The model under review builds one solid part; all positions refer to its coordinate system, in mm. A direction names the side the tool comes from. Round coordinates to 2 decimals unless told otherwise and drop trailing zeros. Write each loop counter-clockwise with the first axis right and the second up, starting at its lowest first coordinate (ties: lowest second). Pieces come first, ordered by that corner, then holes.
Item 1: Add section B-B (z = -13). Give the boundary of the cut face in (x, y), plus the area to 3 significant figures.
Item 2: Clearance check with flat-ended pins moving along their axes: pin 1 Ø3 at (y, z) = (-2.5, 20) entering from -X; pin 2 Ø3 at (x, y) = (-15.5, -4.5) entering from -Z (3 decimals); pin 3 Ø5.5 at (x, z) = (0, -14.29) entering from +Y; pin 4 Ø1.5 at (x, z) = (12, 20) entering from +Y. State where each tip first meets the part, or that it passes through.
Item 3: Machinability: for faces 1 (the face through (-12.7, -3, -8)), 2 (the face through (-6.45, -3, 28)), 3 (the face through (12.7, -3, -8)), 4 (the face through (12.7, -3, 21)), which of the approach directions +Z, -Z, +X, -X, +Y, -Y give a long, thin tool a straight path to every point of the face, cutting with its end or side? Answer none if there is none.
Item 4: Add section A-A (x = 0). Give the boundary of the cut face in (y, z) (1 decimal).
Item 5: Add section D-D (x = -7.5). Give the boundary of the cut face in (y, z) (3 decimals), plus the area to 3 significant figures.
Item 6: To check wall thickness, follow L1, parallel to Z at x = 0, y = -3.85 (1 decimal); L2, parallel to X at y = -4.05, z = 21; L3, parallel to Z at x = -1.5, y = -3.3 (3 decimals). State the ranges of each line that lie inside material, in increasing order.
```python
from build123d import *

# Parameters (mm, degrees)
F0_R     = 3.175
F1_DEPTH = 5.842
F2_R     = 3.175


with BuildPart() as f1:
    # F0 (on Front) → F1 (new body)
    with BuildSketch(Plane.XZ):
        Polygon((-6.45, 25.4), (-12.7, 25.4), (-12.7, 15.875), (-18.542, 15.875), (-18.542, 3.175), (-12.7, 3.175), (-12.7, -6.35), (-12.7, -22.225), (12.7, -22.225), (12.7, -6.35), (12.7, 3.175), (18.542, 3.175), (18.542, 15.875), (12.7, 15.875), (12.7, 25.4), (6.45, 25.4), (6.45, 31.242), (-6.45, 31.242), align=None)
        with Locations((0, -14.2875)):
            Circle(F0_R, mode=Mode.SUBTRACT)
    extrude(amount=F1_DEPTH)

    # F2
    f2_edges = [f1.edges().sort_by_distance(p)[0] for p in [
        (-12.7, -2.921, -22.225),
        (12.7, -2.921, -22.225),
    ]]
    fillet(f2_edges, radius=F2_R)


solid = f1.part
```
Numbers:
1. outline: (-12.7, -5.84) - (-2.9, -5.84) - (-2.9, 0) - (-12.7, 0) - close; (2.9, -5.84) - (12.7, -5.84) - (12.7, 0) - (2.9, 0) - close
1. area: 114 mm2
2. pin 1: stops at x = -12.7
2. pin 2: stops at z = 3.175
2. pin 3: passes through
2. pin 4: stops at y = 0
3. face 1: -Z, -X, +Y, -Y
3. face 2: +Z, -X, +Y, -Y
3. face 3: -Z, +X, +Y, -Y
3. face 4: +Z, +X, +Y, -Y
4. outline: (-5.8, -22.2) - (0, -22.2) - (0, -17.5) - (-5.8, -17.5) - close; (-5.8, -11.1) - (0, -11.1) - (0, 31.2) - (-5.8, 31.2) - close
5. outline: (-5.842, -22.225) - (0, -22.225) - (0, 25.4) - (-5.842, 25.4) - close
5. area: 278 mm2
6. L1: z = -22.2 to -17.5, -11.1 to 31.2
6. L2: x = -12.7 to 12.7
6. L3: z = -22.225 to -17.086, -11.489 to 31.242
